```python
from build123d import *

# Parameters (mm, degrees)
MAINPLATE_DEPTH               = 2
TOPPLATE_W                    = 23
TOPPLATE_H                    = 10
BOSS_EXTRUDE6_DEPTH           = 2
SKETCH7_W                     = 8
SKETCH7_H                     = 0.8
SLOTSFORMETALTABS_DEPTH       = 10
SKETCH8_W                     = 8
SKETCH8_H                     = 4
ACCESSHOLESFORMETALTABS_DEPTH = 1
SKETCH9_W                     = 4
SKETCH9_H                     = 10
CUT_EXTRUDE3_DEPTH            = 0.5
SKETCH10_W                    = 33
SKETCH10_H                    = 0.5
CUT_EXTRUDE4_DEPTH            = 11


with BuildPart() as part:
    # Sketch1 → MainPlate (new body)
    with BuildSketch(Plane.XY):
        with BuildLine():
            Line((0, 0), (54, 0))
            Line((54, 0), (54, 18))
            ThreePointArc((54, 18), (59, 23), (54, 28))
            Line((54, 28), (13, 28))
            Line((13, 28), (3, 12))
            Line((3, 12), (3, 2))
            Line((3, 2), (0, 1))
            Line((0, 1), (0, 0))
        make_face()
    extrude(amount=-MAINPLATE_DEPTH)

    # TopPlate → Boss-Extrude6 (add)
    with BuildSketch(Plane(origin=(0, 28, 0), x_dir=(1, 0, 0), z_dir=(0, 1, 0))):
        with Locations((28.5, 5)):
            Rectangle(TOPPLATE_W, TOPPLATE_H)
    extrude(amount=BOSS_EXTRUDE6_DEPTH)

    # Sketch7 → SlotsForMetalTabs (cut)
    with BuildSketch(Plane.XZ):
        with Locations((49, -1)):
            Rectangle(SKETCH7_W, SKETCH7_H)
        with Locations((29, -1)):
            Rectangle(SKETCH7_W, SKETCH7_H)
    extrude(amount=-SLOTSFORMETALTABS_DEPTH, mode=Mode.SUBTRACT)

    # Sketch8 → AccessHolesForMetalTabs (cut)
    with BuildSketch(Plane.XY):
        with Locations((49, 8)):
            Rectangle(SKETCH8_W, SKETCH8_H)
        with Locations((49, 2)):
            Rectangle(SKETCH8_W, SKETCH8_H)
        with Locations((29, 2)):
            Rectangle(SKETCH8_W, SKETCH8_H)
        with Locations((29, 8)):
            Rectangle(SKETCH8_W, SKETCH8_H)
    extrude(amount=-ACCESSHOLESFORMETALTABS_DEPTH, mode=Mode.SUBTRACT)

    # Sketch9 → Cut-Extrude3 (cut)
    with BuildSketch(Plane.XY):
        with Locations((22, 5)):
            Rectangle(SKETCH9_W, SKETCH9_H)
    extrude(amount=-CUT_EXTRUDE3_DEPTH, mode=Mode.SUBTRACT)

    # Sketch10 → Cut-Extrude4 (cut, through all)
    with BuildSketch(Plane.XY):
        with Locations((36.5, 0.25)):
            Rectangle(SKETCH10_W, SKETCH10_H)
    extrude(amount=-CUT_EXTRUDE4_DEPTH, mode=Mode.SUBTRACT)


solid = part.part
```
Geometry check sheet. Reference: the model listing, model coordinates, mm. A direction names the side the tool comes from. Coordinates: 2 decimals unless noted, no trailing zeros. Order: outer loops, then holes, each group sorted by start corner. A loop starts at its lowest first (then second) coordinate and runs counter-clockwise, first axis right, second up.
Item 1: Section check A-A (x = 28.5). Enter the section's corners in (y, z).
Item 2: Section check C-C (z = -5.75). Enter the section's corners in (x, y), plus the area to 3 significant figures.
Item 3: Section check B-B (x = 47.5). Enter the section's corners in (y, z), plus the area to 3 significant figures.
Item 4: Tool access check on faces 5 (the flat face through (29, 10, -1)), 6 (the flat face through (40, 29, -5)), 7 (the flat face through (33, 5, -1)), 8 (the flat face through (15, 28, -1)), 9 (the flat face through (49, 5, -1.4)). Record the directions out of +Z, -Z, +X, -X, +Y, -Y that give a thin tool (end or side, any length) a straight path to the whole face; none if there is none.
Item 5: Mould release check, pull along Z, two halves, no side actions. Record for faces 1 (the flat face through (29, 5, -1.4)), 2 (the flat face through (29, 14, -2)), 3 (the flat face through (22, 5, -0.5)), 4 (the flat face through (1.5, 1.5, -1)): released by +Z, released by -Z, zero draft, split by the parting line, or undercut.
Item 6: Section check D-D (x = 18). Enter the section's corners in (y, z).
Item 7: Depth check by flat-ended pin: pin 1 (2 mm diameter, centred on x = 28, y = 4.5, fed in from -Z); pin 2 (0.7 mm diameter, centred on x = 47.5, z = -1, fed in from -Y); pin 3 (1 mm diameter, centred on y = 29, z = -6.5, fed in from +X). Enter the tip coordinate at first touch or a pass-through.
Item 8: Scan lines: line 1 along X through (y, z) = (2.5, -1); line 2 along Z through (x, y) = (9, 19.75); line 3 along X through (y, z) = (11.5, -1.5). Record each from-to range of solid material in increasing order.
Check sheet entries:
1. outline: (0.5, -2) - (28, -2) - (28, -10) - (30, -10) - (30, 0) - (10, 0) - (10, -1.4) - (0.5, -1.4) - close; (4, -0.6) - (6, -0.6) - (6, 0) - (4, 0) - close
2. outline: (17, 28) - (40, 28) - (40, 30) - (17, 30) - close
2. area: 46.0 mm2
3. outline: (0.5, -2) - (28, -2) - (28, 0) - (10, 0) - (10, -1.4) - (0.5, -1.4) - close; (4, -0.6) - (6, -0.6) - (6, 0) - (4, 0) - close
3. area: 42.9 mm2
4. face 5: +Z
4. face 6: +Z, -Z, +X, +Y
4. face 7: none
4. face 8: +Z, -Z, -X, +Y
4. face 9: -Y
5. face 1: undercut
5. face 2: released by -Z
5. face 3: released by +Z
5. face 4: zero draft
6. outline: (0, -2) - (28, -2) - (28, -10) - (30, -10) - (30, 0) - (0, 0) - close
7. pin 1: stops at z = -2
7. pin 2: stops at y = 10
7. pin 3: stops at x = 40
8. line 1: x = 3 to 25, 33 to 45, 53 to 54
8. line 2: z = -2 to 0
8. line 3: x = 3 to 54
